Job drawing, mm, ordinate dimensions from the low corner. One solid piece. A direction names the side the tool comes from. Coordinates: 2 decimals unless noted, no trailing zeros. Order: outer loops, then holes, each group sorted by start corner. A loop starts at its lowest first (then second) coordinate and runs counter-clockwise, first axis right, second up. Notation, with made-up numbers: (0, -28.75) - (56, -28.75) arc R24 cw to (56, -7.75) - close; hole circle Ø1 at (16.25, -8.5). An arc over 180 degrees is marked (long way). Return JSON: item names as keys, results as strings.
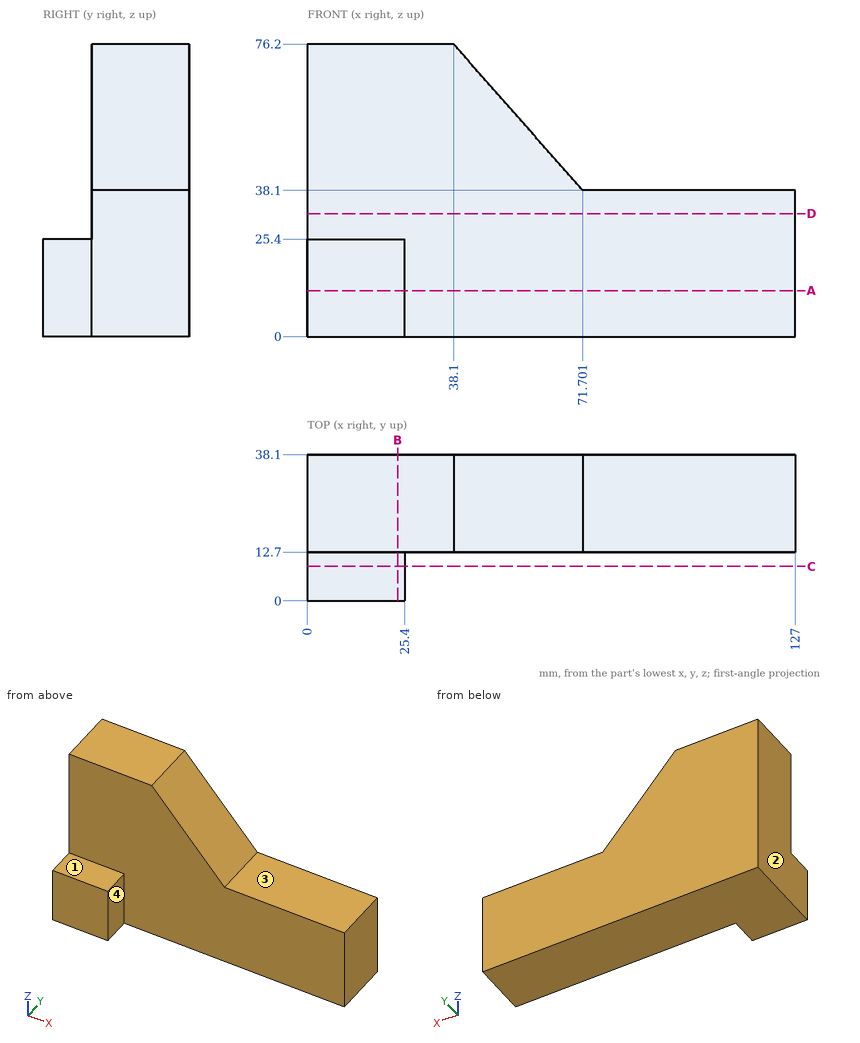
1. Tool access for the marked faces 1, 2, 3 and 4: list every direction of +Z, -Z, +X, -X, +Y, -Y with a clear straight run to the whole face (end or side of a thin tool).
Check values:
{"face 1": "+Z, +X, -X, -Y", "face 2": "+Z, -Z, -X, +Y, -Y", "face 3": "+Z, +X, +Y, -Y", "face 4": "+Z, -Z, +X, -Y"}
2. Cut at A-A on z = 12. Give the cut face in (x, y), plus the area to 3 significant figures.
Check values:
{"outline": "(0, 0) - (25.4, 0) - (25.4, 12.7) - (127, 12.7) - (127, 38.1) - (0, 38.1) - close", "area": "3,550 mm²"}
3. Cut at C-C on y = 9. Give the cut face in (x, z).
Check values:
{"outline": "(0, 0) - (25.4, 0) - (25.4, 25.4) - (0, 25.4) - close"}
4. Probe L1, parallel to Z at x = 76.5, y = 14; L2, parallel to Y at x = 116.5, z = 36.5; L3, parallel to Z at x = 19.5, y = 6.5. List the from-to ranges inside material, lowest first.
Check values:
{"L1": "0 to 38.1", "L2": "12.7 to 38.1", "L3": "0 to 25.4"}
5. Cut at B-B on x = 23.5. Give the cut face in (y, z), plus the area to 3 significant figures.
Check values:
{"outline": "(0, 0) - (38.1, 0) - (38.1, 76.2) - (12.7, 76.2) - (12.7, 25.4) - (0, 25.4) - close", "area": "2,260 mm²"}
6. Cut at D-D on z = 32. Give the cut face in (x, y), plus the area to 3 significant figures.
Check values:
{"outline": "(0, 12.7) - (127, 12.7) - (127, 38.1) - (0, 38.1) - close", "area": "3,230 mm²"}
7. Drop flat-ended pins along their axis: pin 1 (10 mm diameter, centred on x = 12, y = 6.5, fed in from +Z); pin 2 (4 mm diameter, centred on y = 28.5, z = 68.5, fed in from +X); pin 3 (6.5 mm diameter, centred on y = 5.5, z = 19, fed in from +X). Give the stop position or say it passes through.
Check values:
{"pin 1": "z = 25.4", "pin 2": "x = 46.65", "pin 3": "x = 25.4"}
